Build history of the part. All positions in model axes, mm. A direction names the side the tool comes from. Round coordinates to 2 decimals unless told otherwise and drop trailing zeros. Order: outer loops, then holes, each group sorted by start corner. A loop starts at its lowest first (then second) coordinate and runs counter-clockwise, first axis right, second up. Notation, with made-up numbers: (87, 30.25) -> (112, 30.25) arc R12 cw to (112, 34.25) -> close; hole circle Ø6 at (79, 30). An arc over 180 degrees is marked (long way). Answer as a JSON object with one key per item and string values.
from build123d import *

# Parameters (mm, degrees)
SKETCH1_R      = 20.066
SKETCH1_R_2    = 17.526
EXTRUDE1_DEPTH = 44.45
EXTRUDE2_START = -12.7
SKETCH2_R      = 34.925
SKETCH2_R_2    = 17.526
EXTRUDE2_DEPTH = 12.7
SKETCH3_R      = 34.925
SKETCH3_R_2    = 17.526
EXTRUDE3_DEPTH = 12.7


with BuildPart() as part:
    # Sketch1 → Extrude1 (new body)
    with BuildSketch(Plane(origin=(0, 0, 0), x_dir=(1, 0, 0), z_dir=(0, 1, 0))):
        with Locations(Location((0, 0, 0), (0, 0, 270))):
            Circle(SKETCH1_R)
        with Locations(Location((0, 0, 0), (0, 0, 270))):
            Circle(SKETCH1_R_2, mode=Mode.SUBTRACT)
    extrude(amount=EXTRUDE1_DEPTH)

    # Sketch2 → Extrude2 (add)
    with BuildSketch(Plane(origin=(0, 44.45, 0), x_dir=(1, 0, 0), z_dir=(0, 1, 0)).offset(EXTRUDE2_START)):
        with Locations(Location((0, 0, 0), (0, 0, 270))):
            Circle(SKETCH2_R)
        with Locations(Location((0, 0, 0), (0, 0, 270))):
            Circle(SKETCH2_R_2, mode=Mode.SUBTRACT)
    extrude(amount=EXTRUDE2_DEPTH)

    # Sketch3 → Extrude3 (add)
    with BuildSketch(Plane.XZ):
        with Locations(Location((0, 0, 0), (0, 0, 90))):
            Circle(SKETCH3_R)
        with Locations(Location((0, 0, 0), (0, 0, 90))):
            Circle(SKETCH3_R_2, mode=Mode.SUBTRACT)
    extrude(amount=-EXTRUDE3_DEPTH)


solid = part.part
1) Flat gauge pins, fed straight in: pin 1 Ø1.5 at (x, y) = (22, 39.5) entering from +Z; pin 2 Ø4 at (y, z) = (34.5, 14.5) entering from +X; pin 3 Ø2 at (y, z) = (38, -1) entering from +X (3 decimals). Where does each tip first touch, or does it go through?
Checked values:
{"pin 1": "stops at z = 27.72", "pin 2": "stops at x = 32.61", "pin 3": "stops at x = 34.925"}
2) Pull direction Y, two halves, no side cores. Call faces 3 (the face through (-15, 31.75, 15)), 4 (the face through (-8, 0, -16)), 5 (the face through (34.094, 6.261, -7.571)): pulls with the +Y half, pulls with the -Y half, needs draft (parallel to the pull), parting line crosses it, or undercut.
Checked values:
{"face 3": "undercut", "face 4": "pulls with the -Y half", "face 5": "needs draft"}
3) Cut at D-D, the plane z = 22. Give the cut face in (x, y), plus the area to 3 significant figures.
Checked values:
{"outline": "(-27.12, 0) -> (27.12, 0) -> (27.12, 12.7) -> (-27.12, 12.7) -> close; (-27.12, 31.75) -> (27.12, 31.75) -> (27.12, 44.45) -> (-27.12, 44.45) -> close", "area": "1,380 mm²"}
4) Cut at B-B, the plane x = 0. Give the cut face in (y, z) (3 decimals), plus the area to 3 significant figures.
Checked values:
{"outline": "(0, -34.925) -> (12.7, -34.925) -> (12.7, -20.066) -> (31.75, -20.066) -> (31.75, -34.925) -> (44.45, -34.925) -> (44.45, -17.526) -> (0, -17.526) -> close; (0, 17.526) -> (44.45, 17.526) -> (44.45, 34.925) -> (31.75, 34.925) -> (31.75, 20.066) -> (12.7, 20.066) -> (12.7, 34.925) -> (0, 34.925) -> close", "area": "981 mm²"}
5) Probe L1, parallel to X at y = 23, z = 0.5; L2, parallel to Y at x = -22, z = 24; L3, parallel to X at y = 34, z = 0 (3 decimals). List the from-to ranges inside material, lowest first. Write a range as from..to.
Checked values:
{"L1": "x = -20.06..-17.52, 17.52..20.06", "L2": "y = 0..12.7, 31.75..44.45", "L3": "x = -34.925..-17.526, 17.526..34.925"}
6) Cut at C-C, the plane y = 39. Give the cut face in (x, z) (3 decimals).
Checked values:
{"outline": "circle Ø69.85 at (0, 0); hole circle Ø35.052 at (0, 0)"}
7) Cut at A-A, the plane z = 0. Give the cut face in (x, y) (3 decimals).
Checked values:
{"outline": "(-34.925, 0) -> (-17.526, 0) -> (-17.526, 44.45) -> (-34.925, 44.45) -> (-34.925, 31.75) -> (-20.066, 31.75) -> (-20.066, 12.7) -> (-34.925, 12.7) -> close; (17.526, 0) -> (34.925, 0) -> (34.925, 12.7) -> (20.066, 12.7) -> (20.066, 31.75) -> (34.925, 31.75) -> (34.925, 44.45) -> (17.526, 44.45) -> close"}
8) Which spindle directions (+Z, -Z, +X, -X, +Y, -Y) get a long thin tool onto all of the face, cutting with end or side? Do faces 1 (the face through (8, 44.45, -16)), 2 (the face through (-19.6, 22.1, -4.3)). Say none if no direction does.
Checked values:
{"face 1": "+Z, -Z, +X, -X, +Y", "face 2": "none"}
